Autodesk Fusion 360 part; units mm, degrees
sketch "top" plane through (0, 0, 0) normal (0, 0, 1) x (1, 0, 0)
  line L0 (0, 0) -> (68, 0)
  line L1 (68, 0) -> (68, -25)
  line L2 (68, -25) -> (0, -25)
  line L3 (0, -25) -> (0, 0)
  line L4 (70.5, -27.5) -> (-2.5, -27.5)
  line L5 (-2.5, -27.5) -> (-2.5, 2.5)
  line L6 (-2.5, 2.5) -> (70.5, 2.5)
  line L7 (70.5, 2.5) -> (70.5, -27.5)
  dimension "d1" = 68
  dimension "d2" = 25
  dimension "d3" = -2.5
extrude "Extrude1" add sketch "top" along normal blind 3 contours L0 L1 L2 L3 | L4 L5 L6 L7
extrude "Extrude2" add sketch "top" along normal blind 80 from surface at 3
fillet "Fillet1" radius 5 8 edges at (-2.5, -27.5, 41.5) (70.5, -27.5, 41.5) (70.5, 2.5, 41.5) (0, 0, 43) (0, -25, 43) (68, -25, 43) (68, 0, 43) (-2.5, 2.5, 41.5)
sketch "side" plane through (0, 2.5, 0) normal (0, 1, 0) x (-1, 0, 0)
  line L0 (-2.5, 0) -> (-2.5, 83)
  line L1 (-2.5, 83) -> (-65.5, 83)
  line L2 (-65.5, 83) -> (-65.5, 0)
  line L3 (-65.5, 0) -> (-2.5, 0)
  line L4 (-65.5, 0) -> (-65.5, 83)
  line L5 (-2.5, 83) -> (-2.5, 0)
  line L6 (-65.5, 83) -> (-2.5, 83)
  line L7 (-2.5, 0) -> (-65.5, 0)
  line L8 (-34, 83) -> (-34, 0) construction
  line L9 (-57.5, 66.25) -> (-57.5, 16.75)
  arc A0 (-57.5, 16.75) -> (-40, 16.75) centre (-48.75, 16.75) ccw
  line L10 (-40, 16.75) -> (-40, 66.25)
  arc A1 (-40, 66.25) -> (-57.5, 66.25) centre (-48.75, 66.25) ccw
  line L11 (-48.75, 66.25) -> (-48.75, 16.75) construction
  arc A2 (-10.5, 66.25) -> (-28, 66.25) centre (-19.25, 66.25) ccw
  line L12 (-10.5, 66.25) -> (-10.5, 16.75)
  arc A3 (-28, 16.75) -> (-10.5, 16.75) centre (-19.25, 16.75) ccw
  line L13 (-28, 16.75) -> (-28, 66.25)
  circle A4 centre (-48.75, 53) radius 1.5
  circle A5 centre (-19.25, 53) radius 1.5
  dimension "d11" = 8
  dimension "d12" = 6
  dimension "d13" = 8
  dimension "d14" = 8
  dimension "d17" = 3
  dimension "d18" = 30
extrude "Extrude3" cut sketch "side" against normal up to surface (2.5 mm away) contours L9 A0 L10 A1 | A2 L12 A3 L13 | A4 | A5
extrude "Extrude4" cut sketch "side" against normal up to surface (2.5 mm away) from surface at -27.5 contours A4 | A5
For this review, take the finished solid that the model builds, in its own axes (mm). A direction names the side the tool comes from. Round coordinates to 2 decimals unless told otherwise and drop trailing zeros. Loops run counter-clockwise (first coordinate to the right, second up) from the corner with the lowest first, then second, coordinate; pieces in that order, holes last. Notation, with made-up numbers: (-11.5, 68.25) - (43.5, 68.25) arc R19 ccw to (43.5, 85.25) - close; hole circle Ø5 at (22, -40). An arc over 180 degrees is marked (long way). Put each result on its own line as item: value. Start each with the question number.
1. Insertion check: P1, Ø7.5, axis at x = 19, y = -13.5, coming from the +Z side; P2, Ø0.8, axis at y = 1.5, z = 45, coming from the -X side; P3, Ø3, axis at y = 1, z = 41, coming from the +X side; P4, Ø2.5, axis at x = 48.75, z = 53, coming from the +Y side. Each pin has a flat end and moves straight along its axis. Give the tip position at first contact, or say it passes through.
2. For probe 1 along Z at (x, y) = (48.75, -25.9); probe 2 along Y at (x, z) = (33.5, 34.5); probe 3 along X at (y, z) = (-9, 7.5), list the stretches that pass through material, from the lowest coordinate up. Write a range as [from, to].
3. Consider section C-C on z = 31. State the section outline as (x, y) points.
4. For faces 5 (the cylindrical face through (2, -1, 44)), 6 (the flat face through (34, -27.5, 41)), 7 (the flat face through (40, 1, 41)), list the 3-axis set-ups (+Z, -Z, +X, -X, +Y, -Y) from which the entire face can be reached by the end or side of a thin tool; tool diameter is ignored.
5. Consider section D-D on y = -6. State the section outline as (x, z) points.
6. Consider section A-A on x = 48.75. State the section outline as (y, z) points, plus the area to 3 significant figures.
7. Mouldability with a two-part tool opening along Y and no side actions: class faces 1 (the cylindrical face through (69.07, 1, 42.08)), 2 (the flat face through (31, -26, 83)), 3 (the flat face through (34, 0, 42)), 4 (the cylindrical face through (67, -2, 44)) as +Y half, -Y half, draft (parallel to the pull), parting line (faces both ways), or undercut.
8. Consider section B-B on z = 53. State how many separate pieces and enclosed holes the cut face has, plus the area to 4 significant figures.
Result sheet:
1. P1: z = 3
1. P2: x = -0.97
1. P3: x = 70.08
1. P4: through
2. probe 1: [0, 51.5], [54.5, 83]
2. probe 2: [-27.5, -25], [0, 2.5]
2. probe 3: [-2.5, 0], [68, 70.5]
3. outline: (-2.5, -22.5) arc R5 ccw to (2.5, -27.5) - (65.5, -27.5) arc R5 ccw to (70.5, -22.5) - (70.5, -2.5) arc R5 ccw to (65.5, 2.5) - (57.5, 2.5) - (57.5, 0) - (63, 0) arc R5 cw to (68, -5) - (68, -20) arc R5 cw to (63, -25) - (5, -25) arc R5 cw to (0, -20) - (0, -5) arc R5 cw to (5, 0) - (10.5, 0) - (10.5, 2.5) - (2.5, 2.5) arc R5 ccw to (-2.5, -2.5) - close; (28, 0) - (40, 0) - (40, 2.5) - (28, 2.5) - close
4. face 5: +Z
4. face 6: +Z, -Z, +X, -X, -Y
4. face 7: +Y
5. outline: (-2.5, 0) - (70.5, 0) - (70.5, 83) - (68, 83) - (68, 3) - (0, 3) - (0, 83) - (-2.5, 83) - close
6. outline: (-27.5, 0) - (2.5, 0) - (2.5, 8) - (0, 8) - (0, 3) - (-25, 3) - (-25, 51.5) - (-27.5, 51.5) - close; (-27.5, 54.5) - (-25, 54.5) - (-25, 83) - (-27.5, 83) - close; (0, 75) - (2.5, 75) - (2.5, 83) - (0, 83) - close
6. area: 315 mm^2
7. face 1: +Y half
7. face 2: draft
7. face 3: undercut
7. face 4: undercut
8. separate pieces: 4
8. enclosed holes: 0
8. area: 387.5 mm^2
